The drawing under review shows one solid part. Ordinate dimensions are in mm from its lowest x, y, z. A direction names the side the tool comes from. Give positions to 0.01 mm unless a question says otherwise; leave off trailing zeros. Loops run counter-clockwise (first coordinate to the right, second up) from the corner with the lowest first, then second, coordinate; pieces in that order, holes last. Notation, with made-up numbers: (66, 63.25) - (119, 63.25) arc R23 ccw to (119, 88.25) - close; hole circle Ø4 at (43, 2). An arc over 180 degrees is marked (long way). Answer as CSV lines item,"result".
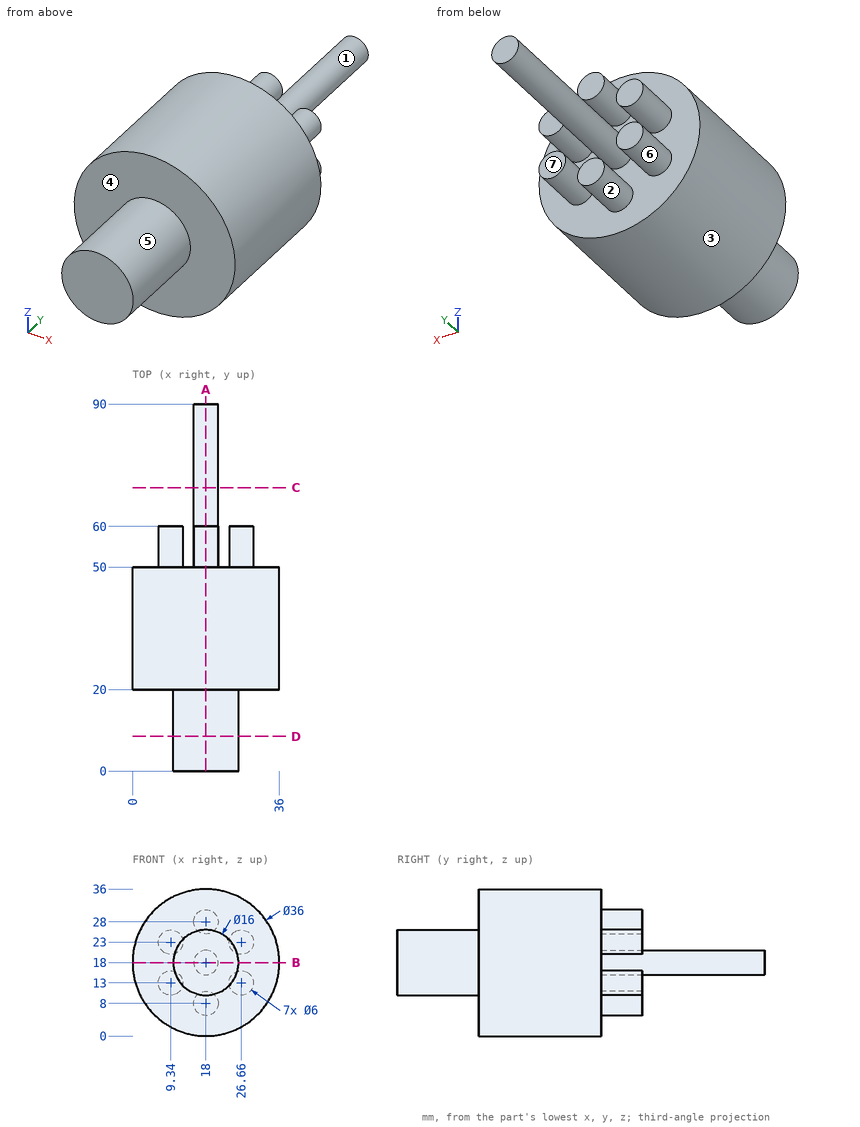
1) Consider section A-A on x = 18. Write out the cut boundary in (y, z), and give its area (3 significant figures).
From the geometry:
outline,"(0, 10) - (20, 10) - (20, 0) - (50, 0) - (50, 5) - (60, 5) - (60, 11) - (50, 11) - (50, 15) - (90, 15) - (90, 21) - (50, 21) - (50, 25) - (60, 25) - (60, 31) - (50, 31) - (50, 36) - (20, 36) - (20, 26) - (0, 26) - close"
area,"1,760 mm^2"
2) Consider section C-C on y = 69.5. Write out the cut boundary in (x, z), and give its area (3 significant figures).
From the geometry:
outline,"circle Ø6 at (18, 18)"
area,"28.3 mm^2"
3) Draft analysis for pull direction Z (two halves, no side actions). For the marked faces 1, 2, 3 and 4, state which applies: pulls with the +Z half, pulls with the -Z half, needs draft (parallel to the pull), parting line crosses it, or undercut.
From the geometry:
face 1,"undercut"
face 2,"undercut"
face 3,"parting line crosses it"
face 4,"needs draft"
4) Wall thickness on line 1 (Y direction, x = 22, z = 16.5); line 2 (Y direction, x = 25, z = 32.5); line 3 (Z direction, x = 20, y = 52) (1 decimal): over which ranges is each line inside the solid? List them lowest first. Write a range as from..to.
From the geometry:
line 1,"y = 0..50"
line 2,"y = 20..50"
line 3,"z = 5.8..10.2, 15.8..20.2, 25.8..30.2"
5) Consider section D-D on y = 8.5. Write out the cut boundary in (x, z), and give its area (3 significant figures).
From the geometry:
outline,"circle Ø16 at (18, 18)"
area,"201 mm^2"
6) Machinability: for the marked faces 5, 6 and 7, which of the approach directions +Z, -Z, +X, -X, +Y, -Y give a long, thin tool a straight path to every point of the face, cutting with its end or side? Answer none if there is none.
From the geometry:
face 5,"-Y"
face 6,"+Y"
face 7,"+Z, -Z, +X, +Y"
7) Insertion check: P1, Ø3, axis at x = 17, z = 27.5, coming from the +Y side; P2, Ø6, axis at x = 17.5, z = 23.5, coming from the +Y side; P3, Ø4, axis at y = 9.5, z = 9, coming from the -X side; P4, Ø4, axis at x = 6, y = 55, coming from the +Z side. Each pin has a flat end and moves straight along its axis. Give the tip position at first contact, or say it passes through.
From the geometry:
P1,"stops at y = 60"
P2,"stops at y = 90"
P3,"stops at x = 14.13"
P4,"stops at z = 25.68"
8) Consider section B-B on z = 18. Write out the cut boundary in (x, y).
From the geometry:
outline,"(0, 20) - (10, 20) - (10, 0) - (26, 0) - (26, 20) - (36, 20) - (36, 50) - (21, 50) - (21, 90) - (15, 90) - (15, 50) - (0, 50) - close"
